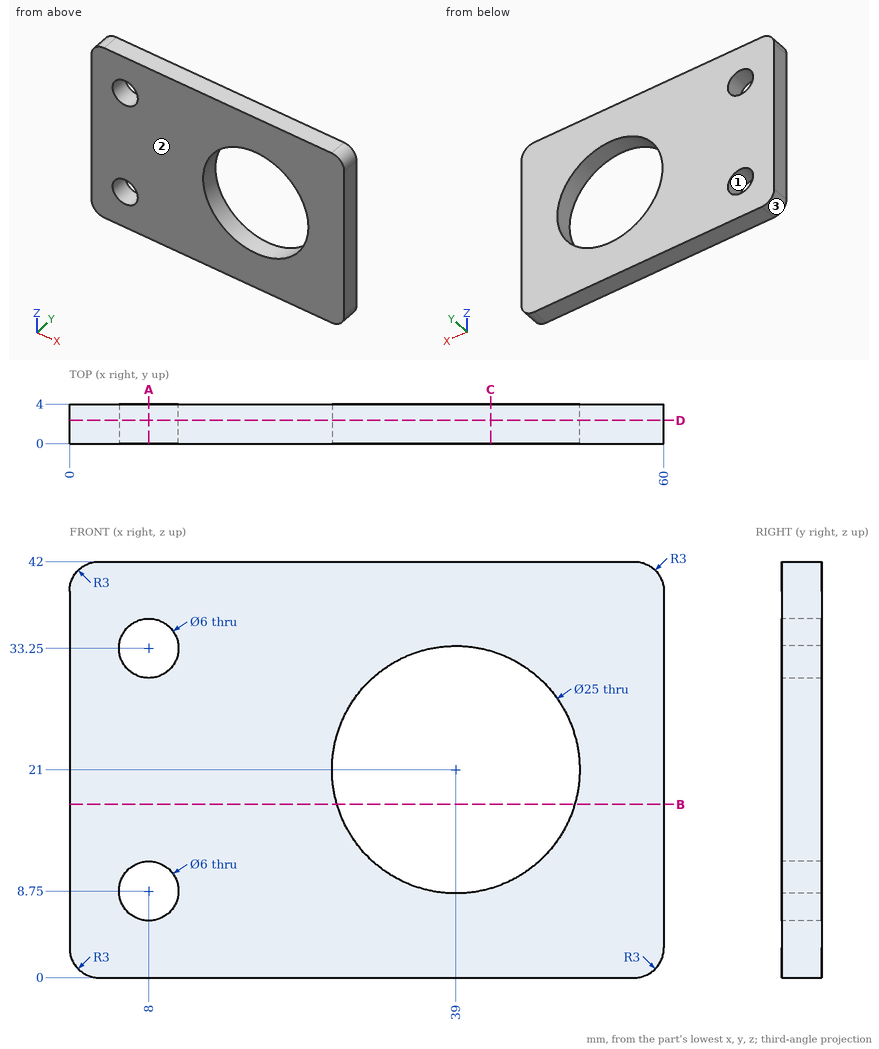
Could you check a few things on this drawing? It's one solid part, dimensions in mm from its lowest x, y, z. Coordinates: 2 decimals unless noted, no trailing zeros. Write each loop counter-clockwise with the first axis right and the second up, starting at its lowest first coordinate (ties: lowest second). Pieces come first, ordered by that corner, then holes. Notation, with made-up numbers: M 59.25,64 L 74.25,64 A10 ccw 74.25,80 Z; hole C 72.25,53 d10. An arc over 180 degrees is marked long. Answer as CSV lines item,"result". Start each with the question number.
Q1. If we mould it in two halves opening along Z, with no side actions, what happens to the marked faces 1, 2 and 3? For each: pulls with the +Z half, pulls with the -Z half, needs draft (parallel to the pull), parting line crosses it, or undercut.
Q2. Suppose I cut it at D-D, the plane y = 2.35. List the corners of the cut face in (x, z) for me.
Q3. Will this pin go through, and if not, where does the flat tip stop? pin 1 Ø5.5 at (x, z) = (8, 33.25) entering from +Y.
Q4. I need wall thicknesses on probe 1 along Z at (x, y) = (8, 2.6); probe 2 along X at (y, z) = (0.8, 9.5); probe 3 along Z at (x, y) = (47, 1.9). Which ranges of each line are inside material? Lowest first, please. Write a range as [from, to].
Q5. Suppose I cut it at A-A, the plane x = 8. List the corners of the cut face in (y, z) for me, then the cut area to 3 significant figures.
Q6. Suppose I cut it at C-C, the plane x = 42.5. List the corners of the cut face in (y, z) for me.
Q7. Suppose I cut it at B-B, the plane z = 17.5. List the corners of the cut face in (x, y) for me, then the cut area to 3 significant figures.
Entries:
1,face 1,"undercut"
1,face 2,"needs draft"
1,face 3,"pulls with the -Z half"
2,outline,"M 0,3 A3 ccw 3,0 L 57,0 A3 ccw 60,3 L 60,39 A3 ccw 57,42 L 3,42 A3 ccw 0,39 Z; hole C 8,8.75 d6; hole C 8,33.25 d6; hole C 39,21 d25"
3,pin 1,"passes through"
4,probe 1,"z = [0, 5.75], [11.75, 30.25], [36.25, 42]"
4,probe 2,"x = [0, 5.1], [10.9, 34.1], [43.9, 60]"
4,probe 3,"z = [0, 11.4], [30.6, 42]"
5,outline,"M 0,0 L 4,0 L 4,5.75 L 0,5.75 Z; M 0,11.75 L 4,11.75 L 4,30.25 L 0,30.25 Z; M 0,36.25 L 4,36.25 L 4,42 L 0,42 Z"
5,area,"120 mm²"
6,outline,"M 0,0 L 4,0 L 4,9 L 0,9 Z; M 0,33 L 4,33 L 4,42 L 0,42 Z"
7,outline,"M 0,0 L 27,0 L 27,4 L 0,4 Z; M 51,0 L 60,0 L 60,4 L 51,4 Z"
7,area,"144 mm²"
